CAD build for the part. Positions are in the model's coordinates, mm. Give positions to 0.01 mm unless a question says otherwise; leave off trailing zeros. Write each loop counter-clockwise with the first axis right and the second up, starting at its lowest first coordinate (ties: lowest second). Pieces come first, ordered by that corner, then holes. Notation, with made-up numbers: (51, 41.25) -> (92, 41.25) arc R18 ccw to (92, 61.25) -> close; hole circle Ø5 at (73.5, 32.5). An arc over 180 degrees is marked (long way). Answer as a JSON object with one key per item and string values.
```python
from build123d import *


with BuildPart() as part:
    # Esboço1 → Revolução1 (revolve)
    with BuildSketch(Plane(origin=(0, 0, 0), x_dir=(0, 0, -1), z_dir=(1, 0, 0)), mode=Mode.PRIVATE) as revolu_o1_sk:
        with BuildLine():
            Line((-1.25, 5), (1.25, 5))
            ThreePointArc((1.25, 5), (1.603553391, 4.853553391), (1.75, 4.5))
            Line((1.75, 4.5), (1.75, 3.5))
            ThreePointArc((1.75, 3.5), (1.603553391, 3.146446609), (1.25, 3))
            Line((1.25, 3), (-1.25, 3))
            ThreePointArc((-1.25, 3), (-1.603553391, 3.146446609), (-1.75, 3.5))
            Line((-1.75, 3.5), (-1.75, 4.5))
            ThreePointArc((-1.75, 4.5), (-1.603553391, 4.853553391), (-1.25, 5))
        make_face()
    revolve(revolu_o1_sk.sketch.rotate(Axis((0, 0, 0), (0, 0, 1)), 90), axis=Axis((0, 0, 0), (0, 0, 1)))


solid = part.part
```
1) Slice it at A-A (x = 0). List the corners of the cut face in (y, z), then the cut area to 3 significant figures.
Model answer:
{"outline": "(-5, -1.25) arc R0.5 ccw to (-4.5, -1.75) -> (-3.5, -1.75) arc R0.5 ccw to (-3, -1.25) -> (-3, 1.25) arc R0.5 ccw to (-3.5, 1.75) -> (-4.5, 1.75) arc R0.5 ccw to (-5, 1.25) -> close; (3, -1.25) arc R0.5 ccw to (3.5, -1.75) -> (4.5, -1.75) arc R0.5 ccw to (5, -1.25) -> (5, 1.25) arc R0.5 ccw to (4.5, 1.75) -> (3.5, 1.75) arc R0.5 ccw to (3, 1.25) -> close", "area": "13.6 mm2"}
2) Wall check: probe 1 along Y at (x, z) = (0, -0.15); probe 2 along X at (y, z) = (-1.75, 1.2); probe 3 along Y at (x, z) = (1.25, 1.55). Give the ranges that are in metal, low to high.
Model answer:
{"probe 1": "y = -5 to -3, 3 to 5", "probe 2": "x = -4.68 to -2.44, 2.44 to 4.68", "probe 3": "y = -4.74 to -2.84, 2.84 to 4.74"}
3) Slice it at D-D (z = 1.4). List the corners of the cut face in (x, y).
Model answer:
{"outline": "circle Ø9.95 at (0, 0); hole circle Ø6.05 at (0, 0)"}
4) Mould opens along Y. For faces 1 (the cylindrical face through (5, 0, 0)), 2 (the flat face through (0, 4, 1.75)), 3 (the cylindrical face through (-2.86, -0.9, 0.02)) say: released by +Y, released by -Y, zero draft, split by the parting line, or undercut.
Model answer:
{"face 1": "split by the parting line", "face 2": "zero draft", "face 3": "undercut"}
5) Pin check, flat tips, straight feed: pin 1 (5 mm diameter, centred on x = 0, y = -1, fed in from +Z); pin 2 (1.5 mm diameter, centred on y = 3, z = -1, fed in from +X); pin 3 (2 mm diameter, centred on y = -2, z = -1, fed in from -X). Stop position of each tip, or through.
Model answer:
{"pin 1": "stops at z = 1.75", "pin 2": "stops at x = 4.47", "pin 3": "stops at x = -4.9"}
6) Slice it at C-C (z = 0.6). List the corners of the cut face in (x, y).
Model answer:
{"outline": "circle Ø10 at (0, 0); hole circle Ø6 at (0, 0)"}
